from build123d import *
from build123d.topology import SkipClean

# Parameters (mm, degrees)
ESBO_O1_R                = 20
RESSALTO_EXTRUS_O1_DEPTH = 4
RESSALTO_EXTRUS_O2_START = -3
ESBO_O2_R                = 3.5
RESSALTO_EXTRUS_O2_DEPTH = 3
RESSALTO_EXTRUS_O4_DEPTH = 35
ESBO_O4_R                = 1.6
CORTE_EXTRUS_O1_DEPTH    = 10
CORTE_EXTRUS_O3_DEPTH    = 8
ESBO_O10_W               = 6.5
ESBO_O10_H               = 10
ESBO_O10_R               = 0.75
ESBO_O10_W_2             = 4.75
RESSALTO_EXTRUS_O5_DEPTH = 4.2


# Read off the part's stored shape, not the designer's step: Ressalto-extrusão4
with BuildPart() as part:
    # Esboço1 → Ressalto-extrusão1 (new body)
    with BuildSketch(Plane.XY):
        Circle(ESBO_O1_R)
        with BuildLine():
            ThreePointArc((-16, -2), (-18, 0), (-16, 2))
            Line((-16, 2), (-0.65053243, 3.439012585))
            ThreePointArc((-0.65053243, 3.439012585), (-0.32669248, 3.484719791), (0, 3.5))
            ThreePointArc((0, 3.5), (0.32669248, 3.484719791), (0.65053243, 3.439012585))
            Line((0.65053243, 3.439012585), (16, 2))
            ThreePointArc((16, 2), (18, 0), (16, -2))
            Line((16, -2), (0.65053243, -3.439012585))
            ThreePointArc((0.65053243, -3.439012585), (0.32669248, -3.484719791), (0, -3.5))
            ThreePointArc((0, -3.5), (-0.32669248, -3.484719791), (-0.65053243, -3.439012585))
            Line((-0.65053243, -3.439012585), (-16, -2))
        make_face(mode=Mode.SUBTRACT)
    extrude(amount=RESSALTO_EXTRUS_O1_DEPTH)

    # Esboço2 → Ressalto-extrusão2 (add)
    with SkipClean():  # the faces are left unmerged after this step: merging them gives an invalid solid
        with BuildSketch(Plane.XY.offset(4).offset(RESSALTO_EXTRUS_O2_START)):
            with BuildLine():
                Line((-19.070572075, 6.026050177), (19.070572075, 6.026050177))
                ThreePointArc((19.070572075, 6.026050177), (20, 0), (19.070572075, -6.026050177))
                Line((19.070572075, -6.026050177), (-19.070572075, -6.026050177))
                ThreePointArc((-19.070572075, -6.026050177), (-20, 0), (-19.070572075, 6.026050177))
            make_face()
            with Locations(Location((0, 0, 0), (0, 0, 100.711650086))):
                Circle(ESBO_O2_R, mode=Mode.SUBTRACT)
        extrude(amount=RESSALTO_EXTRUS_O2_DEPTH)

    # Ressalto-extrusão4 outline → Ressalto-extrusão4 (add)
    with SkipClean():  # the faces are left unmerged after this step: merging them gives an invalid solid
        with BuildSketch(Plane(origin=(0, 0, 0), x_dir=(-1, 0, 0), z_dir=(0, 0, -1))):
            with BuildLine():
                ThreePointArc((3, -19.773719933), (5.026901421, -19.357950876), (7, -18.734993995))
                Line((7, -18.734993995), (7, 18.734993995))
                ThreePointArc((7, 18.734993995), (5.026901421, 19.357950876), (3, 19.773719933))
                Line((3, 19.773719933), (3, -19.773719933))
            make_face()
        extrude(amount=RESSALTO_EXTRUS_O4_DEPTH)

    # Esboço4 → Corte-extrusão1 (cut)
    with SkipClean():  # the faces are left unmerged after this step: merging them gives an invalid solid
        with BuildSketch(Plane(origin=(-3, 0, 0), x_dir=(0, 0, -1), z_dir=(1, 0, 0))):
            with Locations(Location((23, -10.925, 0), (0, 0, 90))):
                Circle(ESBO_O4_R)
            with BuildLine():
                ThreePointArc((17.263269231, 7.868871717), (29.5, 10.925), (17.263269231, 13.981128283))
                ThreePointArc((17.263269231, 13.981128283), (13.35, 10.925), (17.263269231, 7.868871717))
            make_face()
        extrude(amount=-CORTE_EXTRUS_O1_DEPTH, mode=Mode.SUBTRACT)

    # Esboço9 → Corte-extrusão3 (cut)
    with SkipClean():  # the faces are left unmerged after this step: merging them gives an invalid solid
        with BuildSketch(Plane.ZY.offset(7)):
            with BuildLine():
                Line((0, 8), (0, -8))
                ThreePointArc((0, -8), (-8, 0), (0, 8))
            make_face()
        extrude(amount=-CORTE_EXTRUS_O3_DEPTH, mode=Mode.SUBTRACT)

    # Esboço10 → Ressalto-extrusão5 (add)
    # profile 1 of 2: a face of its own
    with SkipClean():  # the faces are left unmerged after this step: merging them gives an invalid solid
        with BuildSketch(Plane.ZY.offset(7)):
            with Locations((-3.25, 10.925)):
                Rectangle(ESBO_O10_W, ESBO_O10_H)
            with Locations(Location((-4.25, 10.925, 0), (0, 0, 270))):
                Circle(ESBO_O10_R, mode=Mode.SUBTRACT)
        # profile 2 of 2: a face of its own
        with BuildSketch(Plane.ZY.offset(7)):
            with Locations((-31.875, 10.925)):
                Rectangle(ESBO_O10_W_2, ESBO_O10_H)
            with Locations(Location((-31.875, 10.925, 0), (0, 0, 270))):
                Circle(ESBO_O10_R, mode=Mode.SUBTRACT)
        extrude(amount=RESSALTO_EXTRUS_O5_DEPTH)


solid = part.part
Can you work these out from the model? Positions are in its coordinate system, mm. A direction names the side the tool comes from. Round coordinates to 2 decimals unless told otherwise and drop trailing zeros. Order: outer loops, then holes, each group sorted by start corner. A loop starts at its lowest first (then second) coordinate and runs counter-clockwise, first axis right, second up. Notation, with made-up numbers: (-1.5, 18) - (24.5, 18) arc R17 cw to (24.5, 49) - close; hole circle Ø8 at (79.25, 29.5). An arc over 180 degrees is marked (long way). Answer in a Markdown table with one row per item.
(1) Suppose I cut it at A-A, the plane z = -24. Please give me the cut outline in (x, y) (3 decimals), plus the area to 3 significant figures.
From the geometry:
| item | result |
|---|---|
| outline | (-7, -18.735) arc R20 ccw to (-3, -19.774) - (-3, -12.174) - (-7, -12.174) - close; (-7, -9.676) - (-3, -9.676) - (-3, 4.502) - (-7, 4.502) - close; (-7, 17.348) - (-3, 17.348) - (-3, 19.774) arc R20 ccw to (-7, 18.735) - close |
| area | 93.3 mm2 |
(2) If we mould it in two halves opening along X, with no side actions, what happens to faces 5 (the face through (8.22, 2.73, 0.49)), 6 (the face through (-7, 7, -2)), 7 (the face through (-9.071, 10.232, -4.537))? For each: released by +X, released by -X, zero draft, split by the parting line, or undercut.
From the geometry:
| item | result |
|---|---|
| face 5 | undercut |
| face 6 | released by +X |
| face 7 | zero draft |
(3) Suppose I cut it at C-C, the plane x = 11. Please give me the cut outline in (y, z), plus the area to 3 significant figures.
From the geometry:
| item | result |
|---|---|
| outline | (-16.7, 0) - (-2.47, 0) - (-2.47, 1) - (2.47, 1) - (2.47, 0) - (16.7, 0) - (16.7, 4) - (-16.7, 4) - close |
| area | 129 mm2 |
(4) For P1, Ø2, axis at x = -9, z = -32.5, coming from the +Y side (3 decimals); P2, Ø1.3, axis at x = -9, z = -32.5, coming from the -Y side (3 decimals); P3, Ø0.8, axis at y = 11, z = -32, coming from the -X side, each with a flat end and sliding along its axis, tell me the tip position at first contact or that it passes through.
From the geometry:
| item | result |
|---|---|
| P1 | stops at y = 15.925 |
| P2 | stops at y = 5.925 |
| P3 | stops at x = -7 |
(5) Which directions (+Z, -Z, +X, -X, +Y, -Y) give clear straight access to the entire face, cutting with the end or side of a thin tool? Please do faces 1 (the face through (-11.2, 11, -33)), 2 (the face through (-18, 0, 0.5)), 3 (the face through (-9, 15.925, -32)), 4 (the face through (-9, 0, 1)).
From the geometry:
| item | result |
|---|---|
| face 1 | -Z, -X, +Y, -Y |
| face 2 | -Z |
| face 3 | -Z, -X, +Y |
| face 4 | none |
